Source: CAD feature listing. Evaluate the final solid. Frame: model axes, mm. A direction names the side the tool comes from. Round coordinates to 2 decimals unless told otherwise and drop trailing zeros. Loops run counter-clockwise (first coordinate to the right, second up) from the corner with the lowest first, then second, coordinate; pieces in that order, holes last. Notation, with made-up numbers: (11.25, 29.5) -> (30.25, 29.5) arc R22 cw to (30.25, 49.5) -> close; hole circle Ø4 at (18.25, 61.25). An arc over 180 degrees is marked (long way). Return JSON: item names as keys, results as strings. Group by question number.
```python
from build123d import *

# Parameters (mm, degrees)
F1_DEPTH = 4
F2_DEPTH = 10
F3_DEPTH = 8.2
F4_W     = 5.5
F4_H     = 33
F4_W_2   = 14.5
F4_H_2   = 5.5
F5_DEPTH = 10


with BuildPart() as f1:
    # F0 (on Top) → F1 (new body)
    with BuildSketch(Plane.XY):
        with BuildLine():
            ThreePointArc((49, -4), (58.8994949366, 0.1005050634), (63, 10))
            Line((63, 10), (63, 114.5))
            ThreePointArc((63, 114.5), (58.8994949366, 124.3994949366), (49, 128.5))
            Line((49, 128.5), (10, 128.5))
            ThreePointArc((10, 128.5), (0.1005050634, 124.3994949366), (-4, 114.5))
            Line((-4, 114.5), (-4, 10))
            ThreePointArc((-4, 10), (0.1005050634, 0.1005050634), (10, -4))
            Line((10, -4), (49, -4))
        make_face()
        with BuildLine():
            Line((49, 0), (10, 0))
            ThreePointArc((10, 0), (2.9289321881, 2.9289321881), (0, 10))
            Line((0, 10), (0, 114.5))
            ThreePointArc((0, 114.5), (2.9289321881, 121.5710678119), (10, 124.5))
            Line((10, 124.5), (49, 124.5))
            ThreePointArc((49, 124.5), (56.0710678119, 121.5710678119), (59, 114.5))
            Line((59, 114.5), (59, 10))
            ThreePointArc((59, 10), (56.0710678119, 2.9289321881), (49, 0))
        make_face(mode=Mode.SUBTRACT)
        with BuildLine():
            ThreePointArc((0, 10), (2.9289321881, 2.9289321881), (10, 0))
            Line((10, 0), (49, 0))
            ThreePointArc((49, 0), (56.0710678119, 2.9289321881), (59, 10))
            Line((59, 10), (59, 114.5))
            ThreePointArc((59, 114.5), (56.0710678119, 121.5710678119), (49, 124.5))
            Line((49, 124.5), (10, 124.5))
            ThreePointArc((10, 124.5), (2.9289321881, 121.5710678119), (0, 114.5))
            Line((0, 114.5), (0, 10))
        make_face()
        with BuildLine():
            ThreePointArc((57.5, 10), (55.0104076401, 3.9895923599), (49, 1.5))
            Line((49, 1.5), (10, 1.5))
            ThreePointArc((10, 1.5), (3.9895923599, 3.9895923599), (1.5, 10))
            Line((1.5, 10), (1.5, 114.5))
            ThreePointArc((1.5, 114.5), (3.9895923599, 120.5104076401), (10, 123))
            Line((10, 123), (49, 123))
            ThreePointArc((49, 123), (55.0104076401, 120.5104076401), (57.5, 114.5))
            Line((57.5, 114.5), (57.5, 10))
        make_face(mode=Mode.SUBTRACT)
        with BuildLine():
            Line((10, 1.5), (49, 1.5))
            ThreePointArc((49, 1.5), (55.0104076401, 3.9895923599), (57.5, 10))
            Line((57.5, 10), (57.5, 114.5))
            ThreePointArc((57.5, 114.5), (55.0104076401, 120.5104076401), (49, 123))
            Line((49, 123), (10, 123))
            ThreePointArc((10, 123), (3.9895923599, 120.5104076401), (1.5, 114.5))
            Line((1.5, 114.5), (1.5, 10))
            ThreePointArc((1.5, 10), (3.9895923599, 3.9895923599), (10, 1.5))
        make_face()
        with BuildLine():
            Line((37.5, 121.5), (51.5, 121.5))
            ThreePointArc((51.5, 121.5), (52.9142135624, 120.9142135624), (53.5, 119.5))
            Line((53.5, 119.5), (53.5, 113.5))
            ThreePointArc((53.5, 113.5), (52.9142135624, 112.0857864376), (51.5, 111.5))
            Line((51.5, 111.5), (37.5, 111.5))
            ThreePointArc((37.5, 111.5), (36.0857864376, 112.0857864376), (35.5, 113.5))
            Line((35.5, 113.5), (35.5, 119.5))
            ThreePointArc((35.5, 119.5), (36.0857864376, 120.9142135624), (37.5, 121.5))
        make_face(mode=Mode.SUBTRACT)
    extrude(amount=-F1_DEPTH)

    # F0 (on Top) → F2 (join)
    with BuildSketch(Plane.XY):
        with BuildLine():
            ThreePointArc((49, -4), (58.8994949366, 0.1005050634), (63, 10))
            Line((63, 10), (63, 114.5))
            ThreePointArc((63, 114.5), (58.8994949366, 124.3994949366), (49, 128.5))
            Line((49, 128.5), (10, 128.5))
            ThreePointArc((10, 128.5), (0.1005050634, 124.3994949366), (-4, 114.5))
            Line((-4, 114.5), (-4, 10))
            ThreePointArc((-4, 10), (0.1005050634, 0.1005050634), (10, -4))
            Line((10, -4), (49, -4))
        make_face()
        with BuildLine():
            Line((49, 0), (10, 0))
            ThreePointArc((10, 0), (2.9289321881, 2.9289321881), (0, 10))
            Line((0, 10), (0, 114.5))
            ThreePointArc((0, 114.5), (2.9289321881, 121.5710678119), (10, 124.5))
            Line((10, 124.5), (49, 124.5))
            ThreePointArc((49, 124.5), (56.0710678119, 121.5710678119), (59, 114.5))
            Line((59, 114.5), (59, 10))
            ThreePointArc((59, 10), (56.0710678119, 2.9289321881), (49, 0))
        make_face(mode=Mode.SUBTRACT)
        with BuildLine():
            ThreePointArc((0, 10), (2.9289321881, 2.9289321881), (10, 0))
            Line((10, 0), (49, 0))
            ThreePointArc((49, 0), (56.0710678119, 2.9289321881), (59, 10))
            Line((59, 10), (59, 114.5))
            ThreePointArc((59, 114.5), (56.0710678119, 121.5710678119), (49, 124.5))
            Line((49, 124.5), (10, 124.5))
            ThreePointArc((10, 124.5), (2.9289321881, 121.5710678119), (0, 114.5))
            Line((0, 114.5), (0, 10))
        make_face()
        with BuildLine():
            ThreePointArc((57.5, 10), (55.0104076401, 3.9895923599), (49, 1.5))
            Line((49, 1.5), (10, 1.5))
            ThreePointArc((10, 1.5), (3.9895923599, 3.9895923599), (1.5, 10))
            Line((1.5, 10), (1.5, 114.5))
            ThreePointArc((1.5, 114.5), (3.9895923599, 120.5104076401), (10, 123))
            Line((10, 123), (49, 123))
            ThreePointArc((49, 123), (55.0104076401, 120.5104076401), (57.5, 114.5))
            Line((57.5, 114.5), (57.5, 10))
        make_face(mode=Mode.SUBTRACT)
    extrude(amount=F2_DEPTH)

    # F0 (on Top) → F3 (cut)
    with BuildSketch(Plane.XY):
        with BuildLine():
            ThreePointArc((0, 10), (2.9289321881, 2.9289321881), (10, 0))
            Line((10, 0), (49, 0))
            ThreePointArc((49, 0), (56.0710678119, 2.9289321881), (59, 10))
            Line((59, 10), (59, 114.5))
            ThreePointArc((59, 114.5), (56.0710678119, 121.5710678119), (49, 124.5))
            Line((49, 124.5), (10, 124.5))
            ThreePointArc((10, 124.5), (2.9289321881, 121.5710678119), (0, 114.5))
            Line((0, 114.5), (0, 10))
        make_face()
        with BuildLine():
            ThreePointArc((57.5, 10), (55.0104076401, 3.9895923599), (49, 1.5))
            Line((49, 1.5), (10, 1.5))
            ThreePointArc((10, 1.5), (3.9895923599, 3.9895923599), (1.5, 10))
            Line((1.5, 10), (1.5, 114.5))
            ThreePointArc((1.5, 114.5), (3.9895923599, 120.5104076401), (10, 123))
            Line((10, 123), (49, 123))
            ThreePointArc((49, 123), (55.0104076401, 120.5104076401), (57.5, 114.5))
            Line((57.5, 114.5), (57.5, 10))
        make_face(mode=Mode.SUBTRACT)
    extrude(amount=F3_DEPTH, mode=Mode.SUBTRACT)

    # F4 (on face) → F5 (cut)
    with BuildSketch(Plane.XY.offset(10)):
        with Locations((-1.25, 94.5)):
            Rectangle(F4_W, F4_H)
        with Locations((41.75, 125.75)):
            Rectangle(F4_W_2, F4_H_2)
        with BuildLine():
            Line((7, 1.5), (7, -3.6747943312))
            ThreePointArc((7, -3.6747943312), (8.4912125127, -3.9184611333), (10, -4))
            Line((10, -4), (49, -4))
            ThreePointArc((49, -4), (50.5087874873, -3.9184611333), (52, -3.6747943312))
            Line((52, -3.6747943312), (52, 1.5))
            Line((52, 1.5), (49, 1.5))
            Line((49, 1.5), (10, 1.5))
            Line((10, 1.5), (7, 1.5))
        make_face()
    extrude(amount=-F5_DEPTH, mode=Mode.SUBTRACT)


solid = f1.part
```
(1) Set-up query: faces 4 (the face through (-2, 78, 5)), 5 (the face through (52, -2, 5)), 6 (the face through (34.5, 126, 5)). Return all of +Z, -Z, +X, -X, +Y, -Y with unobstructed straight access to the full face (end or side cutting, diameter ignored); none if empty.
(2) Cut plane C-C (z = 6.75). Return loops of the section in (x, y).
(3) Ray query, line 1 (X direction, y = 59, z = 3); line 2 (Y direction, x = 41.5, z = -1.25); line 3 (Z direction, x = 36.5, y = 105.5). Return the intervals inside material, ascending.
(4) Cut plane B-B (z = -1.5). Return loops of the section in (x, y), and give its area (3 significant figures).
(5) Cut plane A-A (x = 40.5). Return loops of the section in (y, z), and give its area (3 significant figures).
(6) Mould query, pull axis X, two halves, no side actions, for faces 1 (the face through (15, 124, 10)), 2 (the face through (55.08, 4.06, 9.09)), 3 (the face through (58.8, 0, 2.9)). Classes: released by +X, released by -X, zero draft, split by the parting line, or undercut.
(7) Cut plane D-D (y = 85.5). Return loops of the section in (x, z).
(8) Pin query (flat end, axial travel): pin 1 (1.4 mm diameter, centred on x = 8, z = 9, fed in from -Y); pin 2 (1.6 mm diameter, centred on y = 126.5, z = 3.5, fed in from -X); pin 3 (6.5 mm diameter, centred on x = 23, z = 5, fed in from -Y). Return the tip coordinate at first contact, or that it passes through.
Answers follow:
{
 "1": {"face 4": "+Z, -X", "face 5": "+Z, -Y", "face 6": "+Z, +Y, -Y"},
 "2": {"outline": "(-4, 10) arc R14 ccw to (7, -3.67) -> (7, 0.46) arc R10 cw to (0, 10) -> (0, 78) -> (-4, 78) -> close; (-4, 111) -> (0, 111) -> (0, 114.5) arc R10 cw to (10, 124.5) -> (34.5, 124.5) -> (34.5, 128.5) -> (10, 128.5) arc R14 ccw to (-4, 114.5) -> close; (49, 124.5) arc R10 cw to (59, 114.5) -> (59, 10) arc R10 cw to (52, 0.46) -> (52, -3.67) arc R14 ccw to (63, 10) -> (63, 114.5) arc R14 ccw to (49, 128.5) -> close"},
 "3": {"line 1": "-4 to 0, 59 to 63", "line 2": "-4 to 111.5, 121.5 to 128.5", "line 3": "-4 to 0"},
 "4": {"outline": "(-4, 10) arc R14 ccw to (10, -4) -> (49, -4) arc R14 ccw to (63, 10) -> (63, 114.5) arc R14 ccw to (49, 128.5) -> (10, 128.5) arc R14 ccw to (-4, 114.5) -> close; hole (35.5, 113.5) arc R2 ccw to (37.5, 111.5) -> (51.5, 111.5) arc R2 ccw to (53.5, 113.5) -> (53.5, 119.5) arc R2 ccw to (51.5, 121.5) -> (37.5, 121.5) arc R2 ccw to (35.5, 119.5) -> close", "area": "8,530 mm^2"},
 "5": {"outline": "(-4, -4) -> (111.5, -4) -> (111.5, 0) -> (-4, 0) -> close; (121.5, -4) -> (128.5, -4) -> (128.5, 0) -> (121.5, 0) -> close", "area": "490 mm^2"},
 "6": {"face 1": "zero draft", "face 2": "undercut", "face 3": "released by +X"},
 "7": {"outline": "(-4, -4) -> (63, -4) -> (63, 10) -> (57.5, 10) -> (57.5, 8.2) -> (59, 8.2) -> (59, 0) -> (-4, 0) -> close"},
 "8": {"pin 1": "y = 1.5", "pin 2": "x = 1.6", "pin 3": "y = 123"}
}
